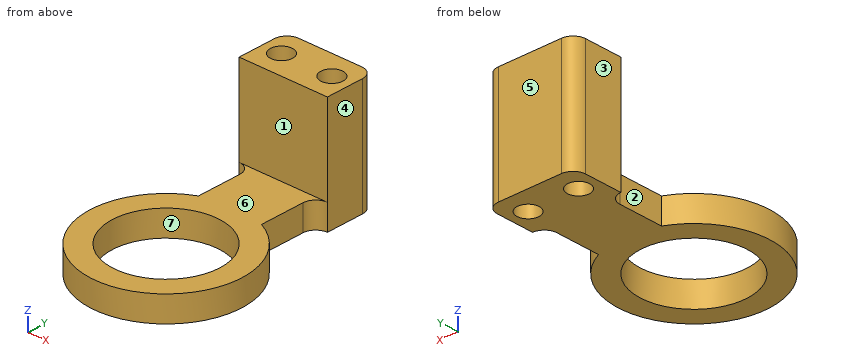
```python
from build123d import *

# Parameters (mm, degrees)
SKETCH_1_W          = 14
SKETCH_1_H          = 8
EXTRUDE_1_DEPTH     = 18
SKETCH_1_3_R        = 8.5
EXTRUDE_2_DEPTH     = 4
FILLET_1_R          = 2
CUT_EXTRUDE_START   = -18
SKETCH_5_R          = 1.75
CUT_EXTRUDE_1_DEPTH = 18
FILLET_3_R          = 2


with BuildPart() as part:
    # 草图1 → 凸台-拉伸1 (new body)
    with BuildSketch(Plane.XY):
        Rectangle(SKETCH_1_W, SKETCH_1_H)
    extrude(amount=EXTRUDE_1_DEPTH)

    # 草图1<3> → 凸台-拉伸2 (add)
    with BuildSketch(Plane.XY):
        with BuildLine():
            Line((5, -13.091287885), (5, -4))
            Line((5, -4), (-5, -4))
            Line((-5, -4), (-5, -13.091287885))
            ThreePointArc((-5, -13.091287885), (0, -36), (5, -13.091287885))
        make_face()
        with Locations((0, -24)):
            Circle(SKETCH_1_3_R, mode=Mode.SUBTRACT)
    extrude(amount=EXTRUDE_2_DEPTH)

    # 圆角1
    fillet_1_edges = [part.edges().sort_by_distance(p)[0] for p in [
        (-5, -4, 2),
        (5, -4, 2),
    ]]
    fillet(fillet_1_edges, radius=FILLET_1_R - 0.0001)  # a hair under: the kernel refuses the full size

    # 草图5 → 切除-拉伸1 (cut)
    with BuildSketch(Plane(origin=(0, 0, 0), x_dir=(-1, 0, 0), z_dir=(0, 0, -1)).offset(CUT_EXTRUDE_START)):
        with Locations((-4, 0)):
            Circle(SKETCH_5_R)
        with Locations(Location((4, 0, 0), (0, 0, 180))):
            Circle(SKETCH_5_R)
    extrude(amount=CUT_EXTRUDE_1_DEPTH, mode=Mode.SUBTRACT)

    # 圆角3
    fillet_3_edges = [part.edges().sort_by_distance(p)[0] for p in [
        (-7, 4, 9),
        (7, 4, 9),
    ]]
    fillet(fillet_3_edges, radius=FILLET_3_R)


solid = part.part
```
Geometry: final body of the model. Coordinates: model frame, mm. Face numbers are marked on the shaded views. A direction names the side the tool comes from. Round coordinates to 2 decimals unless told otherwise and drop trailing zeros. Write each loop counter-clockwise with the first axis right and the second up, starting at its lowest first coordinate (ties: lowest second). Pieces come first, ordered by that corner, then holes. Notation, with made-up numbers: (9, -39.75) -> (50, -39.75) arc R11 cw to (50, -19.75) -> close; hole circle Ø10 at (-1.75, 3.5). An arc over 180 degrees is marked (long way). Return JSON: item names as keys, results as strings.
Q1. Mould query, pull axis Y, two halves, no side actions, for the marked faces 5, 6 and 7. Classes: +Y half, -Y half, draft (parallel to the pull), parting line (faces both ways), or undercut.
From the geometry:
{"face 5": "+Y half", "face 6": "draft", "face 7": "undercut"}
Q2. Section B-B on y = -24. Return the cut outline in (x, z), and give its area (3 significant figures).
From the geometry:
{"outline": "(-12, 0) -> (-8.5, 0) -> (-8.5, 4) -> (-12, 4) -> close; (8.5, 0) -> (12, 0) -> (12, 4) -> (8.5, 4) -> close", "area": "28.0 mm2"}
Q3. Set-up query: the marked faces 1, 2, 3 and 4. Return all of +Z, -Z, +X, -X, +Y, -Y with unobstructed straight access to the full face (end or side cutting, diameter ignored); none if empty.
From the geometry:
{"face 1": "+Z, +X, -X, -Y", "face 2": "+Z, -Z, -X", "face 3": "+Z, -Z, -X, +Y", "face 4": "+Z, -Z, +X, +Y"}
Q4. Section C-C on y = 0. Return the cut outline in (x, z).
From the geometry:
{"outline": "(-7, 0) -> (-5.75, 0) -> (-5.75, 18) -> (-7, 18) -> close; (-2.25, 0) -> (2.25, 0) -> (2.25, 18) -> (-2.25, 18) -> close; (5.75, 0) -> (7, 0) -> (7, 18) -> (5.75, 18) -> close"}
Q5. Ray query, line 1 (Y direction, x = 4, z = 17.25); line 2 (Y direction, x = 0, z = 1.9); line 3 (Y direction, x = -0.5, z = 9). Return the intervals inside material, ascending.
From the geometry:
{"line 1": "-4 to -1.75, 1.75 to 4", "line 2": "-36 to -32.5, -15.5 to 4", "line 3": "-4 to 4"}
Q6. First-contact query: pin 1 Ø3 at (x, y) = (4, -30.5) entering from +Z; pin 2 Ø7 at (x, z) = (-3, 8) entering from -Y; pin 3 Ø1.8 at (y, z) = (-2.5, 7.5) entering from -X; pin 4 Ø3 at (y, z) = (-6.5, 6) entering from +X. Flat tips, straight axial feed; report the tip coordinate or a pass-through.
From the geometry:
{"pin 1": "z = 4", "pin 2": "y = -4", "pin 3": "x = -7", "pin 4": "through"}
Q7. Section A-A on x = 0. Return the cut outline in (y, z), and give its area (3 significant figures).
From the geometry:
{"outline": "(-36, 0) -> (-32.5, 0) -> (-32.5, 4) -> (-36, 4) -> close; (-15.5, 0) -> (4, 0) -> (4, 18) -> (-4, 18) -> (-4, 4) -> (-15.5, 4) -> close", "area": "204 mm2"}
Q8. Section D-D on z = 13. Return the cut outline in (x, y), and give its area (3 significant figures).
From the geometry:
{"outline": "(-7, -4) -> (7, -4) -> (7, 2) arc R2 ccw to (5, 4) -> (-5, 4) arc R2 ccw to (-7, 2) -> close; hole circle Ø3.5 at (-4, 0); hole circle Ø3.5 at (4, 0)", "area": "91.0 mm2"}
